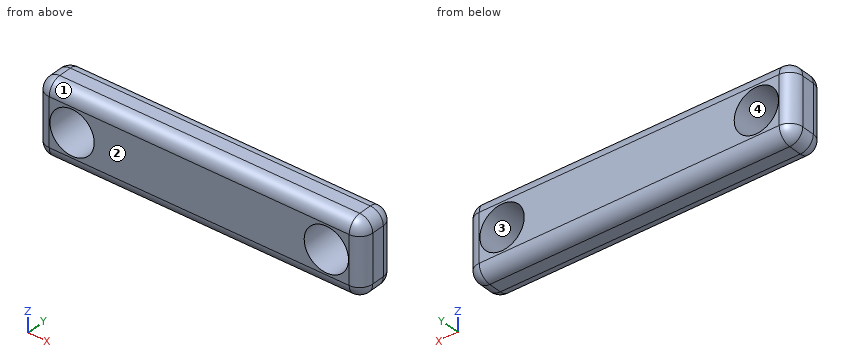
from build123d import *

# Parameters (mm, degrees)
SKETCH1_W           = 25
SKETCH1_H           = 5.7
SKETCH1_R           = 1.7
BOSS_EXTRUDE1_DEPTH = 3
FILLET1_R           = 1


with BuildPart() as part:
    # Sketch1 → Boss-Extrude1 (new body)
    with BuildSketch(Plane(origin=(0, 0, 0), x_dir=(1, 0, 0), z_dir=(0, 1, 0))):
        with Locations((12.5, 2.85)):
            Rectangle(SKETCH1_W, SKETCH1_H)
        with Locations(Location((2.75, 2.85, 0), (0, 0, 270))):
            Circle(SKETCH1_R, mode=Mode.SUBTRACT)
        with Locations(Location((22.25, 2.85, 0), (0, 0, 270))):
            Circle(SKETCH1_R, mode=Mode.SUBTRACT)
    extrude(amount=BOSS_EXTRUDE1_DEPTH)

    # Fillet1
    fillet1_edges = [part.edges().sort_by_distance(p)[0] for p in [
        (25, 3, -2.85),
        (12.5, 3, -5.7),
        (0, 3, -2.85),
        (12.5, 0, -5.7),
        (25, 0, -2.85),
        (12.5, 0, 0),
        (0, 0, -2.85),
        (0, 1.5, -5.7),
        (25, 1.5, -5.7),
        (25, 1.5, 0),
        (0, 1.5, 0),
        (12.5, 3, 0),
    ]]
    fillet(fillet1_edges, radius=FILLET1_R)


solid = part.part
Can you work these out from the model? Positions are in its coordinate system, mm. Face numbers are marked on the shaded views. Give positions to 0.01 mm unless a question says otherwise; leave off trailing zeros. Loops run counter-clockwise (first coordinate to the right, second up) from the corner with the lowest first, then second, coordinate; pieces in that order, holes last. Notation, with made-up numbers: (38, 3.5) - (83, 3.5) arc R6 cw to (83, 7.5) - close; hole circle Ø11 at (-3.5, 7.25). An arc over 180 degrees is marked (long way). One line per item, written item: value.
(1) If we section it at B-B, the plane x = 2.75: List the corners of the cut face in (y, z) for me.
Verdict:
outline: (0, -4.7) arc R1 ccw to (1, -5.7) - (2, -5.7) arc R1 ccw to (3, -4.7) - (3, -4.55) - (0, -4.55) - close; (0, -1.15) - (3, -1.15) - (3, -1) arc R1 ccw to (2, 0) - (1, 0) arc R1 ccw to (0, -1) - close
(2) If we section it at D-D, the plane x = 16: List the corners of the cut face in (y, z) for me.
Verdict:
outline: (0, -4.7) arc R1 ccw to (1, -5.7) - (2, -5.7) arc R1 ccw to (3, -4.7) - (3, -1) arc R1 ccw to (2, 0) - (1, 0) arc R1 ccw to (0, -1) - close
(3) I need wall thicknesses on line 1 along X through (y, z) = (1, -2.85); line 2 along X through (y, z) = (1.7, -3.55); line 3 along Z through (x, y) = (4.25, 2.2). Which ranges of each line are inside material? Lowest first, please.
Verdict:
line 1: 0 to 1.05, 4.45 to 20.55, 23.95 to 25
line 2: 0 to 1.2, 4.3 to 20.7, 23.8 to 25
line 3: -5.68 to -3.65, -2.05 to -0.02
(4) If we section it at A-A, the plane z = -2.85: List the corners of the cut face in (x, y) for me.
Verdict:
outline: (0, 1) arc R1 ccw to (1, 0) - (1.05, 0) - (1.05, 3) - (1, 3) arc R1 ccw to (0, 2) - close; (4.45, 0) - (20.55, 0) - (20.55, 3) - (4.45, 3) - close; (23.95, 0) - (24, 0) arc R1 ccw to (25, 1) - (25, 2) arc R1 ccw to (24, 3) - (23.95, 3) - close
(5) If we section it at C-C, the plane y = 1.25: List the corners of the cut face in (x, z) for me.
Verdict:
outline: (0, -4.7) arc R1 ccw to (1, -5.7) - (24, -5.7) arc R1 ccw to (25, -4.7) - (25, -1) arc R1 ccw to (24, 0) - (1, 0) arc R1 ccw to (0, -1) - close; hole circle Ø3.4 at (2.75, -2.85); hole circle Ø3.4 at (22.25, -2.85)
(6) If we mould it in two halves opening along Z, with no side actions, what happens to the marked faces 1, 2, 3 and 4? For each: released by +Z, released by -Z, zero draft, split by the parting line, or undercut.
Verdict:
face 1: released by +Z
face 2: zero draft
face 3: undercut
face 4: undercut
(7) I'm going to push a flat-ended pin straight in: pin 1 (2 mm diameter, centred on x = 2.75, z = -2.85, fed in from +Y). Where does the tip first touch, or does it pass through?
Verdict:
pin 1: through
